The drawing under review shows one solid part. Ordinate dimensions are in mm from its lowest x, y, z. Give positions to 0.01 mm unless a question says otherwise; leave off trailing zeros. Loops run counter-clockwise (first coordinate to the right, second up) from the corner with the lowest first, then second, coordinate; pieces in that order, holes last. Notation, with made-up numbers: M -38.5,-11.5 L -6.5,-11.5 A9 ccw -6.5,-6.5 Z; hole C -24,80.25 d3. An arc over 180 degrees is marked long. One line per item, written item: value. Start each with the question number.
Q1. We need section B-B on x = 259.5. Write out the cut boundary in (y, z).
Q2. We need section A-A on y = 1.25. Give the number of separate pieces and of enclosed holes in the cut face, plus the area to 3 significant figures.
Q3. To check wall thickness, follow line 1 along Z through (x, y) = (191.5, 3.35); line 2 along Z through (x, y) = (274, 3.5); line 3 along X through (y, z) = (1.35, 53). State the ranges of each line that lie inside material, in increasing order. Write a range as from..to.
Q4. For pin 1 (2.5 mm diameter, centred on y = 3, z = 19, fed in from -X); pin 2 (2.5 mm diameter, centred on x = 39.5, y = 1.5, fed in from -Z); pin 3 (2.5 mm diameter, centred on y = 3, z = 269.5, fed in from +X); pin 4 (2.5 mm diameter, centred on x = 191.5, z = 54, fed in from +Y), all flat-tipped, find the tip position at first contact; note any pin that passes through.
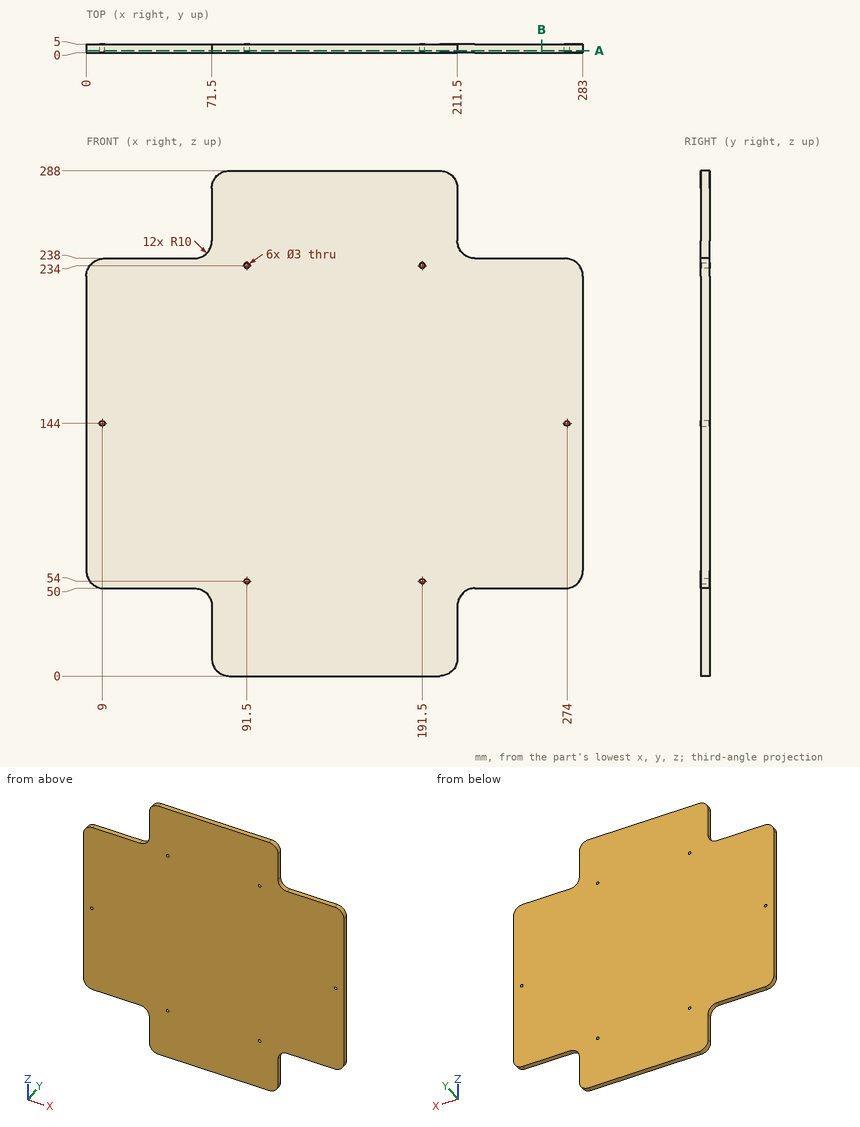
Solved:
1. outline: M 0,50 L 5,50 L 5,238 L 0,238 Z
2. separate pieces: 1
2. enclosed holes: 6
2. area: 67,100 mm2
3. line 1: 0..52.5, 55.5..232.5, 235.5..288
3. line 2: 50.05..142.5, 145.5..237.95
3. line 3: 2.86..90.38, 92.62..190.38, 192.62..280.14
4. pin 1: x = 71.5
4. pin 2: z = 50
4. pin 3: x = 211.5
4. pin 4: through
